Model file for the job. Use its own axes, mm. A direction names the side the tool comes from. Round coordinates to 2 decimals unless told otherwise and drop trailing zeros. Order: outer loops, then holes, each group sorted by start corner. A loop starts at its lowest first (then second) coordinate and runs counter-clockwise, first axis right, second up. Notation, with made-up numbers: (-16, -26) -> (31, -26) arc R33 ccw to (31, 12) -> close; hole circle Ø6 at (33, 32). An arc over 180 degrees is marked (long way). Use CSV: the item, a comma, the result in double quotes.
```python
from build123d import *

# Parameters (mm, degrees)
SKETCH1_W           = 250
SKETCH1_H           = 250
EXTRUDE1_DEPTH      = 30
EXTRUDE2_DEPTH      = 30
FILLET1_R           = 5
FILLET2_R           = 5
SKETCH14_R          = 15
CUT_EXTRUDE1_DEPTH  = 30
SKETCH16_R          = 5.416442209
BOSS_EXTRUDE4_DEPTH = 30
SKETCH17_R          = 15
CUT_EXTRUDE2_DEPTH  = 30


with BuildPart() as part:
    # Sketch1 → Extrude1 (new body)
    with BuildSketch(Plane(origin=(0, 0, 0), x_dir=(1, 0, 0), z_dir=(0, 1, 0))):
        Rectangle(SKETCH1_W, SKETCH1_H)
    extrude(amount=EXTRUDE1_DEPTH)

    # Sketch3 → Extrude2 (add)
    with BuildSketch(Plane(origin=(0, 0, -125), x_dir=(-1, 0, 0), z_dir=(0, 0, -1))):
        with BuildLine():
            Line((-125, 30), (-18.673100048, 307.163472244))
            ThreePointArc((-18.673100048, 307.163472244), (0, 320), (18.673100048, 307.163472244))
            Line((18.673100048, 307.163472244), (125, 30))
            Line((125, 30), (-125, 30))
        make_face()
    extrude(amount=-EXTRUDE2_DEPTH)

    # Fillet1
    fillet1_edges = [part.edges().sort_by_distance(p)[0] for p in [
        (0, 30, -95),
    ]]
    fillet(fillet1_edges, radius=FILLET1_R)

    # Fillet2
    fillet2_edges = [part.edges().sort_by_distance(p)[0] for p in [
        (-125, 15, 125),
        (125, 15, 125),
    ]]
    fillet(fillet2_edges, radius=FILLET2_R)

    # Sketch14 → Cut-Extrude1 (cut)
    with BuildSketch(Plane.XY.offset(-95)):
        with Locations((0.050224631, 153.429955133)):
            Circle(SKETCH14_R)
        with Locations((-0.186934905, 283.429955133)):
            Circle(SKETCH14_R)
    extrude(amount=-CUT_EXTRUDE1_DEPTH, mode=Mode.SUBTRACT)

    # Sketch16 → Boss-Extrude4 (add)
    with BuildSketch(Plane(origin=(-1.938008544, 0, -95), x_dir=(1, 0, 0), z_dir=(0, 0, 1))):
        with Locations((1.836864398, 213.31214362)):
            Circle(SKETCH16_R)
    extrude(amount=-BOSS_EXTRUDE4_DEPTH)

    # Sketch17 → Cut-Extrude2 (cut)
    with BuildSketch(Plane(origin=(0, 30, 0), x_dir=(1, 0, 0), z_dir=(0, 1, 0))):
        with Locations((0, -84.507674079)):
            Circle(SKETCH17_R)
    extrude(amount=-CUT_EXTRUDE2_DEPTH, mode=Mode.SUBTRACT)


solid = part.part
```
Q1. Probe line 1 along Z through (x, y) = (0, 16.5); line 2 along Z through (x, y) = (-25.5, 53); line 3 along Y through (x, z) = (-7.5, 28). List the from-to ranges inside material, lowest first.
From the geometry:
line 1,"z = -125 to 69.51, 99.51 to 125"
line 2,"z = -125 to -95"
line 3,"y = 0 to 30"
Q2. Which spindle directions (+Z, -Z, +X, -X, +Y, -Y) get a long thin tool onto all of the face, cutting with end or side? Do faces 4 (the cylindrical face through (-3.439, 268.787, -109.79)), 5 (the flat face through (-2, 116, -95)). Say none if no direction does.
From the geometry:
face 4,"+Z, -Z"
face 5,"+Z, +X, -X, +Y"
Q3. Cut at A-A (x = 0). Give the cut face in (y, z).
From the geometry:
outline,"(0, -125) -> (138.43, -125) -> (138.43, -95) -> (35, -95) arc R5 cw to (30, -90) -> (30, 69.51) -> (0, 69.51) -> close; (0, 99.51) -> (30, 99.51) -> (30, 125) -> (0, 125) -> close; (168.43, -125) -> (268.43, -125) -> (268.43, -95) -> (168.43, -95) -> close; (298.43, -125) -> (320, -125) -> (320, -95) -> (298.43, -95) -> close"
Q4. Pin check, flat tips, straight feed: pin 1 (5 mm diameter, centred on x = -12.5, z = -76.5, fed in from +Y); pin 2 (12 mm diameter, centred on x = -3, y = 120.5, fed in from +Z). Stop position of each tip, or through.
From the geometry:
pin 1,"stops at y = 30"
pin 2,"stops at z = -95"
Q5. Cut at C-C (z = -99.5). Give the cut face in (x, y).
From the geometry:
outline,"(-125, 0) -> (125, 0) -> (125, 30) -> (18.67, 307.16) arc R20 ccw to (-18.67, 307.16) -> (-125, 30) -> close; hole circle Ø30 at (-0.19, 283.43); hole circle Ø30 at (0.05, 153.43)"
Q6. Mould opens along X. For faces 1 (the flat face through (125, 15, -1)), 2 (the flat face through (-2, 30, 16)), 3 (the cylindrical face through (-3.201, 138.787, -109.79)) say: +X half, -X half, draft (parallel to the pull), parting line (faces both ways), or undercut.
From the geometry:
face 1,"+X half"
face 2,"draft"
face 3,"undercut"
Q7. Cut at B-B (y = 287.5). Give the cut face in (x, z), plus the area to 3 significant figures.
From the geometry:
outline,"(-26.22, -125) -> (-14.62, -125) -> (-14.62, -95) -> (-26.22, -95) -> close; (14.25, -125) -> (26.22, -125) -> (26.22, -95) -> (14.25, -95) -> close"
area,"707 mm²"
Q8. Cut at D-D (x = 81). Give the cut face in (y, z).
From the geometry:
outline,"(0, -125) -> (144.7, -125) -> (144.7, -95) -> (35, -95) arc R5 cw to (30, -90) -> (30, 125) -> (0, 125) -> close"
